from build123d import *

# Parameters (mm, degrees)
CHAMFER1_SIZE  = 0.3
CHAMFER1_SIZE2 = 3.429015691
FILLET1_R      = 0.5


with BuildPart() as part:
    # Sketch3 → Revolve1 (revolve)
    with BuildSketch(Plane.XY, mode=Mode.PRIVATE) as revolve1_sk:
        with BuildLine():
            Line((0, 0), (-5.5, 0))
            Line((-5.5, 0), (-5.5, 8))
            Line((-5.5, 8), (-3.175, 8))
            Line((-3.175, 8), (-3.175, 6))
            ThreePointArc((-3.175, 6), (-3.675, 5.5), (-3.175, 5))
            Line((-3.175, 5), (-3.175, 1.483219346))
            Line((-3.175, 1.483219346), (0, 1.483219346))
            Line((0, 1.483219346), (0, 0))
        make_face()
    revolve(revolve1_sk.sketch.rotate(Axis((0, 0, 0), (0, 1, 0)), 270), axis=Axis((0, 0, 0), (0, 1, 0)))

    # Chamfer1
    chamfer1_edges = [part.edges().sort_by_distance(p)[0] for p in [
        (0, 1.483219346, 3.175),
    ]]
    chamfer1_side = [part.faces().sort_by_distance(p)[0] for p in [
        (0, 1.483219346, 0),
    ]]
    chamfer(chamfer1_edges, length=CHAMFER1_SIZE, length2=CHAMFER1_SIZE2, reference=chamfer1_side[0])

    # Fillet1
    fillet1_edges = [part.edges().sort_by_distance(p)[0] for p in [
        (0, 0, 5.5),
        (0, 8, 5.5),
        (0, 8, 3.175),
    ]]
    fillet(fillet1_edges, radius=FILLET1_R)


solid = part.part
Design review of the part built by this model. Coordinates are the model's own, in mm. A direction names the side the tool comes from. Give positions to 0.01 mm unless a question says otherwise; leave off trailing zeros. Write each loop counter-clockwise with the first axis right and the second up, starting at its lowest first coordinate (ties: lowest second). Pieces come first, ordered by that corner, then holes. Notation, with made-up numbers: M 30,-8.75 L 49,-8.75 A12 cw 49,10.25 Z; hole C 41.25,77 d10. An arc over 180 degrees is marked long. Answer as a JSON object with one key per item and string values. Group by question number.
1) We need section A-A (x = 0). Give the boundary of the cut face in (y, z) (3 decimals), and give its area (3 significant figures).
2) We need section C-C (y = 6.75). Give the boundary of the cut face in (x, z) (3 decimals).
3) We need section D-D (y = 1.25). Give the boundary of the cut face in (x, z), and give its area (3 significant figures).
4) Tool access review of faces 1 (the face through (1.93, 6.74, 2.52)), 2 (the face through (0, 0, 0)): name each direction out of +Z, -Z, +X, -X, +Y, -Y from which nothing blocks a thin tool from reaching the whole face with its end or side.
5) Mouldability with a two-part tool opening along Z and no side actions: class faces 3 (the face through (5.37, 4.05, 1.19)), 4 (the face through (-3, 8, 3)), 5 (the face through (-0.899, 2.841, -2.856)) as released by +Z, released by -Z, zero draft, split by the parting line, or undercut.
6) We need section B-B (z = 0). Give the boundary of the cut face in (x, y) (3 decimals), and give its area (3 significant figures).
7) Clearance check with flat-ended pins moving along their axes: pin 1 Ø1 at (y, z) = (3, -2) entering from -X; pin 2 Ø2 at (x, y) = (-4, 3) entering from -Z; pin 3 Ø5 at (x, z) = (0, 0) entering from +Y; pin 4 Ø6.5 at (x, z) = (-0.5, 0) entering from +Y. State where each tip first meets the part, or that it passes through.
8) For line 1 along X through (y, z) = (6.5, 0) (3 decimals); line 2 along Y through (x, z) = (-2, -0.5); line 3 along Z through (x, y) = (2, 7.75), list the stretches that pass through material, from the lowest coordinate up.
Answer key:
{
 "1": {"outline": "M 0,-5 A0.5 ccw 0.5,-5.5 L 7.5,-5.5 A0.5 ccw 8,-5 L 8,-3.675 A0.5 ccw 7.5,-3.175 L 6,-3.175 A0.5 cw 5,-3.175 L 4.912,-3.175 L 1.483,-2.875 L 1.483,2.875 L 4.912,3.175 L 5,3.175 A0.5 cw 6,3.175 L 7.5,3.175 A0.5 ccw 8,3.675 L 8,5 A0.5 ccw 7.5,5.5 L 0.5,5.5 A0.5 ccw 0,5 Z", "area": "46.5 mm²"},
 "2": {"outline": "C 0,0 d11; hole C 0,0 d6.35"},
 "3": {"outline": "C 0,0 d11", "area": "95.0 mm²"},
 "4": {"face 1": "+Y", "face 2": "+Z, -Z, +X, -X, -Y"},
 "5": {"face 3": "split by the parting line", "face 4": "zero draft", "face 5": "undercut"},
 "6": {"outline": "M -5.5,0.5 A0.5 ccw -5,0 L 5,0 A0.5 ccw 5.5,0.5 L 5.5,7.5 A0.5 ccw 5,8 L 3.675,8 A0.5 ccw 3.175,7.5 L 3.175,6 A0.5 cw 3.175,5 L 3.175,4.912 L 2.875,1.483 L -2.875,1.483 L -3.175,4.912 L -3.175,5 A0.5 cw -3.175,6 L -3.175,7.5 A0.5 ccw -3.675,8 L -5,8 A0.5 ccw -5.5,7.5 Z", "area": "46.5 mm²"},
 "7": {"pin 1": "stops at x = -5.29", "pin 2": "stops at z = -4.61", "pin 3": "stops at y = 1.48", "pin 4": "stops at y = 8"},
 "8": {"line 1": "x = -5.5 to -3.175, 3.175 to 5.5", "line 2": "y = 0 to 1.48", "line 3": "z = -5.05 to -2.55, 2.55 to 5.05"}
}
